```python
from build123d import *

# Parameters (mm, degrees)
SKETCH1_W                              = 96
SKETCH1_H                              = 63.5
MOUNT_BLOCK_DEPTH                      = 6.35
LINEAR_STAGE_4_40_TAPPED_HOLE_D        = 2.2606
OPTICAL_TABLE_1_4_0_25_DIAMETER_HOLE_D = 6.35
OPTICAL_TASBLE_CUT_EXTRUDE_DEPTH       = 6.35


with BuildPart() as part:
    # Sketch1 → Mount Block (new body)
    with BuildSketch(Plane(origin=(0, 0, 0), x_dir=(1, 0, 0), z_dir=(0, 1, 0))):
        Rectangle(SKETCH1_W, SKETCH1_H)
    extrude(amount=MOUNT_BLOCK_DEPTH)

    # Linear Stage #4-40 Tapped Hole (through all)
    with Locations(Plane(origin=(0, 6.35, 0), x_dir=(1, 0, 0), z_dir=(0, 1, 0))):
        with Locations((-27.5, 8.5), (27.618, 8.5), (27.618, -8.518), (-27.5, -8.518)):
            Hole(LINEAR_STAGE_4_40_TAPPED_HOLE_D / 2)

    # Optical Table 1/4 (0.25) Diameter Hole (through all)
    with Locations(Plane(origin=(0, 6.35, 0), x_dir=(1, 0, 0), z_dir=(0, 1, 0))):
        with Locations((-38.1, 25.4), (38.1, 25.4), (38.1, -25.4), (-38.1, -25.4)):
            Hole(OPTICAL_TABLE_1_4_0_25_DIAMETER_HOLE_D / 2)

    # Sketch6 → Optical Tasble Cut-Extrude (cut)
    with BuildSketch(Plane(origin=(0, 6.35, 0), x_dir=(1, 0, 0), z_dir=(0, 1, 0))):
        with BuildLine():
            Line((-34.7218, 25.4), (-34.7218, 17.78))
            ThreePointArc((-34.7218, 17.78), (-38.1, 14.4018), (-41.4782, 17.78))
            Line((-41.4782, 17.78), (-41.4782, 25.4))
            ThreePointArc((-41.4782, 25.4), (-38.1, 28.7782), (-34.7218, 25.4))
        make_face()
        with BuildLine():
            Line((41.4782, 25.4), (41.4782, 17.78))
            ThreePointArc((41.4782, 17.78), (38.1, 14.4018), (34.7218, 17.78))
            Line((34.7218, 17.78), (34.7218, 25.4))
            ThreePointArc((34.7218, 25.4), (38.1, 28.7782), (41.4782, 25.4))
        make_face()
        with BuildLine():
            Line((41.4782, -17.78), (41.4782, -25.4))
            ThreePointArc((41.4782, -25.4), (38.1, -28.7782), (34.7218, -25.4))
            Line((34.7218, -25.4), (34.7218, -17.78))
            ThreePointArc((34.7218, -17.78), (38.1, -14.4018), (41.4782, -17.78))
        make_face()
        with BuildLine():
            Line((-34.7218, -17.78), (-34.7218, -25.4))
            ThreePointArc((-34.7218, -25.4), (-38.1, -28.7782), (-41.4782, -25.4))
            Line((-41.4782, -25.4), (-41.4782, -17.78))
            ThreePointArc((-41.4782, -17.78), (-38.1, -14.4018), (-34.7218, -17.78))
        make_face()
    extrude(amount=-OPTICAL_TASBLE_CUT_EXTRUDE_DEPTH, mode=Mode.SUBTRACT)


solid = part.part
```
Read the model definition and answer for the solid it produces. Units are mm, in the model's axes. A direction names the side the tool comes from. Give positions to 0.01 mm unless a question says otherwise; leave off trailing zeros. Write each loop counter-clockwise with the first axis right and the second up, starting at its lowest first coordinate (ties: lowest second). Pieces come first, ordered by that corner, then holes. Notation, with made-up numbers: M -21.75,-13 L 28.25,-13 A25 ccw 28.25,22 Z; hole C -1.75,12.25 d5. An arc over 180 degrees is marked long. Put each result on its own line as item: value. Start each with the question number.
1. Which of the six approach directions +Z, -Z, +X, -X, +Y, -Y give full straight-line access (tool end or side, diameter ignored) to faces 1 (the flat face through (-1, 3, 31.75)), 2 (the cylindrical face through (-38.174, 3.219, 14.403))?
2. For a pull along X with two mould halves and no side action, classify faces 3 (the cylindrical face through (28.747, 3.131, -8.55)), 4 (the flat face through (48, 3, 0)), 5 (the flat face through (-48, 3, 0)) as released by +X, released by -X, zero draft, split by the parting line, or undercut.
3. Consider line 1 along X through (y, z) = (3, -8.5); line 2 along X through (y, z) = (3.5, 19.5); line 3 along Z through (x, y) = (-38.5, 2.25). Determine where each line is inside the solid, lowest interval first.
4. The part is cut by section A-A, the plane x = -27.5. Give the vertices of the cut face in (y, z).
5. The part is cut by section B-B, the plane z = -8.5. Give the vertices of the cut face in (x, y).
6. This flat-tipped pin is pushed along its axis until it touches: pin 1 Ø1.4 at (x, z) = (27.618, -8.5) entering from -Y. Where does it stop, or does it pass through?
Final values:
1. face 1: +Z, +X, -X, +Y, -Y
1. face 2: +Y, -Y
2. face 3: undercut
2. face 4: released by +X
2. face 5: released by -X
3. line 1: x = -48 to -28.63, -26.37 to 26.49, 28.75 to 48
3. line 2: x = -48 to -41.48, -34.72 to 34.72, 41.48 to 48
3. line 3: z = -31.75 to -28.75, -14.43 to 14.43, 28.75 to 31.75
4. outline: M 0,-31.75 L 6.35,-31.75 L 6.35,-9.63 L 0,-9.63 Z; M 0,-7.37 L 6.35,-7.37 L 6.35,7.39 L 0,7.39 Z; M 0,9.65 L 6.35,9.65 L 6.35,31.75 L 0,31.75 Z
5. outline: M -48,0 L -28.63,0 L -28.63,6.35 L -48,6.35 Z; M -26.37,0 L 26.49,0 L 26.49,6.35 L -26.37,6.35 Z; M 28.75,0 L 48,0 L 48,6.35 L 28.75,6.35 Z
6. pin 1: passes through
